Work out the finished part from the listing and answer in its coordinate system (mm). A direction names the side the tool comes from. Round coordinates to 2 decimals unless told otherwise and drop trailing zeros. Write each loop counter-clockwise with the first axis right and the second up, starting at its lowest first coordinate (ties: lowest second). Pieces come first, ordered by that corner, then holes. Notation, with made-up numbers: M 63,6.25 L 105,6.25 A31 cw 105,30.25 Z; hole C 26.25,22.25 d4. An arc over 180 degrees is marked long. Answer in a Markdown table with one row per item.
Autodesk Inventor part; units mm, degrees
ref_plane "YZ Plane" through (0, 0, 0) normal (1, 0, 0) x (0, 1, 0)
ref_plane "XZ Plane" through (0, 0, 0) normal (0, 1, 0) x (-1, 0, 0)
ref_plane "XY Plane" through (0, 0, 0) normal (0, 0, 1) x (1, 0, 0)
sketch "Sketch1" plane through (0, 0, 0) normal (0, 1, 0) x (-1, 0, 0)
  arc A0 (0, -10.9) -> (0, 10.9) centre (0, 0) ccw
  line L0 (0, -10.9) -> (-30, -10.9)
  line L1 (-30, -10.9) -> (-30, 10.9)
  line L2 (-30, 10.9) -> (0, 10.9)
  line L3 (0, 10.9) -> (0, -10.9) construction
  dimension "d2" = 10.9
  dimension "d3" = 30
  dimension "d4" = 30
  dimension "d5" = 21.8
extrude "Extrusion1" add sketch "Sketch1" along normal blind 1.7
sketch "Sketch2" plane through (0, 1.7, 0) normal (0, 1, 0) x (1, 0, 0)
  arc A0 (0, 10.9) -> (0, -10.9) centre (0, 0) ccw
  circle A1 centre (0, 0) radius 1.5
  dimension "d8" = 3
extrude "Extrusion2" cut sketch "Sketch2" against normal blind 1.7
sketch "Sketch3" plane through (0, 1.7, 0) normal (0, 1, 0) x (1, 0, 0)
  line L0 (30, 10.9) -> (0, 10.9)
  line L1 (0, -10.9) -> (30, -10.9)
  line L2 (30, 10.9) -> (28.3, 10.9)
  line L3 (28.3, 10.9) -> (28.3, -10.9)
  line L4 (28.3, -10.9) -> (30, -10.9)
  line L5 (30, -10.9) -> (30, 10.9)
  point P0 (0, 0)
  dimension "d11" = 1.7
extrude "Extrusion3" add sketch "Sketch3" along normal blind 10
sketch "Sketch4" plane through (28.3, 1.7, -10.9) normal (-1, 0, 0) x (0, 0, 1)
  circle A0 centre (4.4, 5) radius 1.5
  circle A1 centre (17.4, 5) radius 1.5
  line L0 (0, 10) -> (21.8, 10)
  line L1 (21.8, 0) -> (21.8, 10)
  point P0 (10.9, -1.7)
  dimension "d14" = 3
  dimension "d15" = 3
  dimension "d16" = 13
  dimension "d17" = 0
  dimension "d18" = 5
  dimension "d19" = 4.4
extrude "Extrusion4" cut sketch "Sketch4" against normal blind 10
equation "\"BendRadius\" = Thickness"
equation "\"BendReliefWidth\" = Thickness"
equation "\"BendReliefDepth\" = 0.5 * Thickness"
equation "\"CornerReliefSize\" = 4 * Thickness"
equation "\"MinimumRemnant\" = 2 * Thickness"
equation "\"TransitionRadius\" = BendRadius"
equation "\"JacobiRadiusSize\" = BendRadius"
equation "\"GapSize\" = Thickness"
properties part number "A3P3"
1. Determine the mould class of faces 3 (the cylindrical face through (-10.9, 0.8, 0.2)), 4 (the cylindrical face through (29.1, 5.8, -7.7)), 5 (the cylindrical face through (-1.5, 0.86, -0.07)), 6 (the flat face through (9, 1.7, 0)) for opening direction Z: released by +Z, released by -Z, zero draft, split by the parting line, or undercut.
Calculated:
| item | result |
|---|---|
| face 3 | split by the parting line |
| face 4 | undercut |
| face 5 | undercut |
| face 6 | zero draft |
2. The part is cut by section D-D (z = 6). Determine the outline of the cut face in (x, y), plus the area to 3 significant figures.
Calculated:
| item | result |
|---|---|
| outline | M -9.1,0 L 30,0 L 30,5.29 L 28.3,5.29 L 28.3,1.7 L -9.1,1.7 Z; M 28.3,8.11 L 30,8.11 L 30,11.7 L 28.3,11.7 Z |
| area | 78.7 mm² |
3. A tool of negligible diameter and unlimited length cuts with its end or side. For faces 1 (the flat face through (30, 6, 0)), 2 (the flat face through (28.3, 7, 0)), from which of +Z, -Z, +X, -X, +Y, -Y can it reach the whole face along a straight path? Write none if from no direction.
Calculated:
| item | result |
|---|---|
| face 1 | +Z, -Z, +X, +Y, -Y |
| face 2 | +Z, -Z, -X, +Y |
4. The part is cut by section B-B (z = -7). Determine the outline of the cut face in (x, y).
Calculated:
| item | result |
|---|---|
| outline | M -8.36,0 L 30,0 L 30,5.29 L 28.3,5.29 L 28.3,1.7 L -8.36,1.7 Z; M 28.3,8.11 L 30,8.11 L 30,11.7 L 28.3,11.7 Z |
5. Given pin 1 (3.5 mm diameter, centred on y = 6.7, z = -6.5, fed in from +X); pin 2 (6 mm diameter, centred on y = 2.5, z = -5, fed in from -X); pin 3 (4 mm diameter, centred on x = 0, z = 0, fed in from +Y); pin 4 (1.5 mm diameter, centred on y = 7, z = 1.5, fed in from -X), each flat-ended and moving along its own axis, determine where each tip first touches the part or whether it passes through.
Calculated:
| item | result |
|---|---|
| pin 1 | stops at x = 30 |
| pin 2 | stops at x = -10.69 |
| pin 3 | stops at y = 1.7 |
| pin 4 | stops at x = 28.3 |
6. The part is cut by section C-C (x = 13). Determine the outline of the cut face in (y, z).
Calculated:
| item | result |
|---|---|
| outline | M 0,-10.9 L 1.7,-10.9 L 1.7,10.9 L 0,10.9 Z |
7. Consider line 1 along X through (y, z) = (0.85, 0); line 2 along Y through (x, z) = (28.95, -6.5); line 3 along Z through (x, y) = (0, 1.05). Determine where each line is inside the solid, lowest interval first. Write a range as from..to.
Calculated:
| item | result |
|---|---|
| line 1 | x = -10.9..-1.5, 1.5..30 |
| line 2 | y = 0..5.2, 8.2..11.7 |
| line 3 | z = -10.9..-1.5, 1.5..10.9 |
8. The part is cut by section A-A (x = -0.5). Determine the outline of the cut face in (y, z).
Calculated:
| item | result |
|---|---|
| outline | M 0,-10.89 L 1.7,-10.89 L 1.7,-1.41 L 0,-1.41 Z; M 0,1.41 L 1.7,1.41 L 1.7,10.89 L 0,10.89 Z |
